from build123d import *

# Parameters (mm, degrees)
SKETCH1_W               = 281.36
SKETCH1_H               = 30
BOSS_EXTRUDE1_DEPTH     = 3.18
CUT_EXTRUDE1_REACH      = 143.513
SKETCH2_R               = 1.425
MIRROR2_COPY_1_REACH    = 143.513
MIRROR2_COPY_1_SKETCH_R = 1.425
SKETCH3_W               = 275
SKETCH3_H               = 3.19
CUT_EXTRUDE2_DEPTH      = 3.18
SKETCH4_W               = 3.18
SKETCH4_H               = 281.36
BOSS_EXTRUDE2_DEPTH     = 12


with BuildPart() as part:
    # Sketch1 → Boss-Extrude1 (new body)
    with BuildSketch(Plane(origin=(0, 0, 0), x_dir=(0, 0, -1), z_dir=(1, 0, 0))):
        Rectangle(SKETCH1_W, SKETCH1_H)
    extrude(amount=BOSS_EXTRUDE1_DEPTH)

    # Sketch2 → Cut-Extrude1 (cut, up to next)
    with BuildSketch(Plane.ZY, mode=Mode.PRIVATE) as cut_extrude1_sk1:
        with Locations((-127.5, 10)):
            Circle(SKETCH2_R)
    cut_extrude1_tool1 = extrude(cut_extrude1_sk1.sketch, amount=-CUT_EXTRUDE1_REACH, mode=Mode.PRIVATE) & part.part
    # Sketch2 → Cut-Extrude1 (cut, up to next)
    with BuildSketch(Plane.ZY, mode=Mode.PRIVATE) as cut_extrude1_sk2:
        with Locations((-47.91, 10)):
            Circle(SKETCH2_R)
    cut_extrude1_tool2 = extrude(cut_extrude1_sk2.sketch, amount=-CUT_EXTRUDE1_REACH, mode=Mode.PRIVATE) & part.part
    cut_extrude1_1 = cut_extrude1_tool1.solids().sort_by_distance((0, 10, -127.5))[0]
    add(cut_extrude1_1, mode=Mode.SUBTRACT)
    cut_extrude1_2 = cut_extrude1_tool2.solids().sort_by_distance((0, 10, -47.91))[0]
    add(cut_extrude1_2, mode=Mode.SUBTRACT)
    cut_extrude1 = cut_extrude1_1 + cut_extrude1_2  # Cut-Extrude1 as one shape, for the pattern or mirror that repeats it

    # Mirror1: Cut-Extrude1 across plane
    add(cut_extrude1.mirror(Plane.ZX), mode=Mode.SUBTRACT)

    # Mirror2: Cut-Extrude1 across plane
    add(cut_extrude1.mirror(Plane.XY), mode=Mode.SUBTRACT)

    # Mirror2 copy 1 sketch → Mirror2 copy 1 (cut, up to next)
    with BuildSketch(Plane(origin=(0, 0, 0), x_dir=(0, 0, -1), z_dir=(-1, 0, 0)), mode=Mode.PRIVATE) as mirror2_copy_1_sk1:
        with Locations((-127.5, 10)):
            Circle(MIRROR2_COPY_1_SKETCH_R)
    mirror2_copy_1_tool1 = extrude(mirror2_copy_1_sk1.sketch, amount=-MIRROR2_COPY_1_REACH, mode=Mode.PRIVATE) & part.part
    # Mirror2 copy 1 sketch → Mirror2 copy 1 (cut, up to next)
    with BuildSketch(Plane(origin=(0, 0, 0), x_dir=(0, 0, -1), z_dir=(-1, 0, 0)), mode=Mode.PRIVATE) as mirror2_copy_1_sk2:
        with Locations((-47.91, 10)):
            Circle(MIRROR2_COPY_1_SKETCH_R)
    mirror2_copy_1_tool2 = extrude(mirror2_copy_1_sk2.sketch, amount=-MIRROR2_COPY_1_REACH, mode=Mode.PRIVATE) & part.part
    add(mirror2_copy_1_tool1.solids().sort_by_distance((0, -10, 127.5))[0], mode=Mode.SUBTRACT)
    add(mirror2_copy_1_tool2.solids().sort_by_distance((0, -10, 47.91))[0], mode=Mode.SUBTRACT)

    # Sketch3 → Cut-Extrude2 (cut)
    with BuildSketch(Plane(origin=(3.18, 0, 0), x_dir=(0, 0, -1), z_dir=(1, 0, 0))):
        with Locations((0, -1.615)):
            Rectangle(SKETCH3_W, SKETCH3_H)
    extrude(amount=-CUT_EXTRUDE2_DEPTH, mode=Mode.SUBTRACT)

    # Sketch4 → Boss-Extrude2 (add)
    with BuildSketch(Plane.XZ.offset(15)):
        with Locations((1.59, 0)):
            Rectangle(SKETCH4_W, SKETCH4_H)
    extrude(amount=BOSS_EXTRUDE2_DEPTH)


solid = part.part
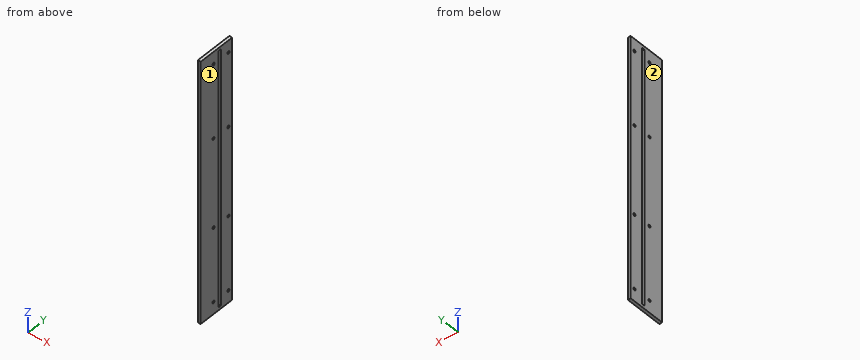
Check sheet for the modelled part. Datum: model origin and axes. Units: mm. Face numbers are marked on the shaded views. Give positions to 0.01 mm unless a question says otherwise; leave off trailing zeros. Write each loop counter-clockwise with the first axis right and the second up, starting at its lowest first coordinate (ties: lowest second). Pieces come first, ordered by that corner, then holes. Notation, with made-up numbers: (-22.75, 34.5) -> (18.25, 34.5) arc R4 cw to (18.25, 38.5) -> close; hole circle Ø5 at (-11.5, -33). An arc over 180 degrees is marked (long way). Write item = value, one per line.
Item 1: Scan lines: probe 1 along Y at (x, z) = (2.35, -127.5) (3 decimals); probe 2 along Y at (x, z) = (2.5, -35); probe 3 along Z at (x, y) = (1.55, -10) (3 decimals). Record each from-to range of solid material in increasing order. Write a range as from..to.
Output:
probe_1 = -27..-11.425, -8.575..-3.21, -0.02..8.575, 11.425..15
probe_2 = -27..-3.21, -0.02..15
probe_3 = -140.68..-128.925, -126.075..-49.335, -46.485..46.485, 49.335..126.075, 128.925..140.68
Item 2: Gauge pin test, flat end, axial feed: pin 1 (3.5 mm diameter, centred on y = 10, z = -127.5, fed in from -X). Record the tip position at first contact, or that the pin passes through.
Output:
pin_1 = 0
Item 3: Release check for a two-part mould opening along X. For the marked faces 1 and 2 record: +X half, -X half, draft (parallel to the pull), parting line (faces both ways), or undercut.
Output:
face_1 = +X half
face_2 = -X half
Item 4: Sectioned sample at B-B on x = 2.55. Count the separate pieces of the cut face and the enclosed holes in it, and give its area (3 significant figures).
Output:
separate_pieces = 1
enclosed_holes = 9
area = 10,900 mm^2
Item 5: Sectioned sample at A-A on z = 120.5. Record the boundary of the cut face in (x, y).
Output:
outline = (0, -27) -> (3.18, -27) -> (3.18, -3.21) -> (0, -3.21) -> close; (0, -0.02) -> (3.18, -0.02) -> (3.18, 15) -> (0, 15) -> close
